Geometry: final body of the model. Coordinates: model frame, mm. Round coordinates to 2 decimals unless told otherwise and drop trailing zeros. Loops run counter-clockwise (first coordinate to the right, second up) from the corner with the lowest first, then second, coordinate; pieces in that order, holes last. Notation, with made-up numbers: M -8.75,-40 L -4.75,-40 A22 cw -4.75,-21 Z; hole C 74.25,28.25 d5. An arc over 180 degrees is marked long. Answer as a JSON object with one key per item and string values.
```python
from build123d import *

# Parameters (mm, degrees)
F0_R     = 4.05
F0_R_2   = 3.200001
F0_R_3   = 3.15
F0_R_4   = 0.75
F0_R_5   = 1
F0_R_6   = 1.1
F1_DEPTH = 2


# Not quite as in the source:
# - ends of sketch curves that miss each other by under 0.0002 mm in the source are joined


with BuildPart() as f1:
    # F0 (on Front) → F1 (new body)
    with BuildSketch(Plane.XZ):
        Polygon((-30.3, -61.250013), (-30.3, -64.250012), (30.300001, -64.250012), (30.300001, 64.250011), (-30.3, 64.250011), align=None)
        with BuildLine():
            ThreePointArc((-23.600001, -59.750013), (-22.7999995588, -59.550011), (-21.9999982215, -59.7500134152))
            Line((-21.9999982215, -59.7500134152), (-21.100001, -59.750013))
            ThreePointArc((-21.100001, -59.750013), (-20.5, -61.2500126379), (-21.1000001998, -62.7500108097))
            Line((-21.1000001998, -62.7500108097), (-21.999999, -62.750012))
            ThreePointArc((-21.999999, -62.750012), (-22.7999995588, -62.950014), (-23.600001, -62.750012))
            Line((-23.600001, -62.750012), (-24.499999, -62.750012))
            ThreePointArc((-24.499999, -62.750012), (-25.1, -61.2500126379), (-24.4999988252, -59.7500141665))
            Line((-24.4999988252, -59.7500141665), (-23.600001, -59.750013))
        make_face(mode=Mode.SUBTRACT)
        with Locations((-19.800001, -47.249931)):
            Circle(F0_R, mode=Mode.SUBTRACT)
        with Locations((-19.800052, -32.249984)):
            Circle(F0_R, mode=Mode.SUBTRACT)
        with Locations((-7.100001, -47.249931)):
            Circle(F0_R, mode=Mode.SUBTRACT)
        with Locations((-7.100052, -32.249984)):
            Circle(F0_R, mode=Mode.SUBTRACT)
        with Locations((-20.549999, -17.249989)):
            Circle(F0_R_2, mode=Mode.SUBTRACT)
        with Locations((-20.549999, -1.999989)):
            Circle(F0_R_3, mode=Mode.SUBTRACT)
        with Locations((-13.8, -22.749991)):
            Circle(F0_R_4, mode=Mode.SUBTRACT)
        with Locations((-7.100052, -17.249986)):
            Circle(F0_R, mode=Mode.SUBTRACT)
        with Locations((-13.200001, -9.499989)):
            Circle(F0_R_5, mode=Mode.SUBTRACT)
        with Locations((-7.100001, -0.749989)):
            Circle(F0_R_2, mode=Mode.SUBTRACT)
        with Locations((7.099976, -47.249957)):
            Circle(F0_R, mode=Mode.SUBTRACT)
        with Locations((7.09995, -32.249928)):
            Circle(F0_R, mode=Mode.SUBTRACT)
        with BuildLine():
            ThreePointArc((22.119986, -59.750023), (22.9199874412, -59.550021), (23.7199887785, -59.7500234152))
            Line((23.7199887785, -59.7500234152), (24.619987, -59.750023))
            ThreePointArc((24.619987, -59.750023), (25.219987, -61.250023), (24.6199863008, -62.7500213341))
            Line((24.6199863008, -62.7500213341), (23.719988, -62.750022))
            ThreePointArc((23.719988, -62.750022), (22.9199874412, -62.950024), (22.119986, -62.750022))
            Line((22.119986, -62.750022), (21.219988, -62.750022))
            ThreePointArc((21.219988, -62.750022), (20.619987, -61.250023), (21.2199901249, -59.7500221189))
            Line((21.2199901249, -59.7500221189), (22.119986, -59.750023))
        make_face(mode=Mode.SUBTRACT)
        with Locations((19.799976, -47.249957)):
            Circle(F0_R, mode=Mode.SUBTRACT)
        with Locations((19.79995, -32.249928)):
            Circle(F0_R, mode=Mode.SUBTRACT)
        with Locations((7.099925, -17.249928)):
            Circle(F0_R, mode=Mode.SUBTRACT)
        with Locations((13.799975, -22.749991)):
            Circle(F0_R_4, mode=Mode.SUBTRACT)
        with Locations((7.100052, -0.749989)):
            Circle(F0_R_2, mode=Mode.SUBTRACT)
        with Locations((13.199999, -9.499989)):
            Circle(F0_R_5, mode=Mode.SUBTRACT)
        with Locations((20.549974, -17.249989)):
            Circle(F0_R_2, mode=Mode.SUBTRACT)
        with Locations((20.549974, -1.999989)):
            Circle(F0_R_3, mode=Mode.SUBTRACT)
        with BuildLine():
            Line((-21.3, 13.150011), (-21.3, 30.750012))
            Line((-21.3, 30.750012), (-21.3, 48.350012))
            ThreePointArc((-21.3, 48.350012), (-21.0363968102, 48.9864088102), (-20.4, 49.250013))
            Line((-20.4, 49.250013), (-19.700001, 49.250013))
            ThreePointArc((-19.700001, 49.250013), (-19.0636041898, 48.9864088102), (-18.8, 48.350012))
            Line((-18.8, 48.350012), (-18.8, 30.750012))
            Line((-18.8, 30.750012), (-18.8, 13.150011))
            ThreePointArc((-18.8, 13.150011), (-19.0636041898, 12.5136141898), (-19.700001, 12.25001))
            Line((-19.700001, 12.25001), (-20.4, 12.250011))
            ThreePointArc((-20.4, 12.250011), (-21.0363968102, 12.5136141898), (-21.3, 13.150011))
        make_face(mode=Mode.SUBTRACT)
        with BuildLine():
            Line((-8.55, 13.150011), (-8.55, 30.750012))
            Line((-8.55, 30.750012), (-8.55, 48.350012))
            ThreePointArc((-8.55, 48.350012), (-8.2863968102, 48.9864088102), (-7.65, 49.250013))
            Line((-7.65, 49.250013), (-6.950001, 49.250013))
            ThreePointArc((-6.950001, 49.250013), (-6.3136041898, 48.9864088102), (-6.05, 48.350012))
            Line((-6.05, 48.350012), (-6.05, 30.750012))
            Line((-6.05, 30.750012), (-6.05, 13.150011))
            ThreePointArc((-6.05, 13.150011), (-6.3136041898, 12.5136141898), (-6.950001, 12.25001))
            Line((-6.950001, 12.25001), (-7.65, 12.250011))
            ThreePointArc((-7.65, 12.250011), (-8.2863968102, 12.5136141898), (-8.55, 13.150011))
        make_face(mode=Mode.SUBTRACT)
        with BuildLine():
            ThreePointArc((-23.600014, 62.750001), (-22.8000125588, 62.950003), (-22.0000112215, 62.7500005848))
            Line((-22.0000112215, 62.7500005848), (-21.100013, 62.750001))
            ThreePointArc((-21.100013, 62.750001), (-20.500013, 61.2500013621), (-21.1000131998, 59.7500031903))
            Line((-21.1000131998, 59.7500031903), (-22.000012, 59.750002))
            ThreePointArc((-22.000012, 59.750002), (-22.8000125588, 59.55), (-23.600014, 59.750002))
            Line((-23.600014, 59.750002), (-24.500012, 59.750002))
            ThreePointArc((-24.500012, 59.750002), (-25.100013, 61.2500013621), (-24.5000093757, 62.7500024055))
            Line((-24.5000093757, 62.7500024055), (-23.600014, 62.750001))
        make_face(mode=Mode.SUBTRACT)
        with Locations((-20.049998, 51.250011)):
            Circle(F0_R_6, mode=Mode.SUBTRACT)
        with BuildLine():
            Line((6.050001, 13.150011), (6.050001, 30.750012))
            Line((6.050001, 30.750012), (6.050001, 48.350012))
            ThreePointArc((6.050001, 48.350012), (6.3136051898, 48.9864088102), (6.950002, 49.250013))
            Line((6.950002, 49.250013), (7.65, 49.250013))
            ThreePointArc((7.65, 49.250013), (8.2863968102, 48.9864088102), (8.550001, 48.350012))
            Line((8.550001, 48.350012), (8.550001, 30.750012))
            Line((8.550001, 30.750012), (8.550001, 13.150011))
            ThreePointArc((8.550001, 13.150011), (8.2863968102, 12.5136141898), (7.65, 12.25001))
            Line((7.65, 12.25001), (6.950002, 12.250011))
            ThreePointArc((6.950002, 12.250011), (6.3136051898, 12.5136141898), (6.050001, 13.150011))
        make_face(mode=Mode.SUBTRACT)
        with BuildLine():
            Line((18.800001, 13.150009), (18.800001, 30.750009))
            Line((18.800001, 30.750009), (18.800001, 48.35001))
            ThreePointArc((18.800001, 48.35001), (19.0636041898, 48.9864068102), (19.700001, 49.250011))
            Line((19.700001, 49.250011), (20.4, 49.25001))
            ThreePointArc((20.4, 49.25001), (21.0363968102, 48.9864068102), (21.300001, 48.35001))
            Line((21.300001, 48.35001), (21.300001, 30.750009))
            Line((21.300001, 30.750009), (21.300001, 13.150009))
            ThreePointArc((21.300001, 13.150009), (21.0363968102, 12.5136121898), (20.4, 12.250008))
            Line((20.4, 12.250008), (19.700001, 12.250008))
            ThreePointArc((19.700001, 12.250008), (19.0636041898, 12.5136121898), (18.800001, 13.150009))
        make_face(mode=Mode.SUBTRACT)
        with Locations((20.050001, 51.250009)):
            Circle(F0_R_6, mode=Mode.SUBTRACT)
        with BuildLine():
            Line((22.119986, 59.750002), (21.219988, 59.750002))
            ThreePointArc((21.219988, 59.750002), (20.619987, 61.2500013621), (21.2199906243, 62.7500024055))
            Line((21.2199906243, 62.7500024055), (22.119986, 62.750001))
            ThreePointArc((22.119986, 62.750001), (22.9199874412, 62.950003), (23.7199887785, 62.7500005848))
            Line((23.7199887785, 62.7500005848), (24.619987, 62.750001))
            ThreePointArc((24.619987, 62.750001), (25.219987, 61.2500013621), (24.6199868002, 59.7500031903))
            Line((24.6199868002, 59.7500031903), (23.719988, 59.750002))
            ThreePointArc((23.719988, 59.750002), (22.9199874412, 59.55), (22.119986, 59.750002))
        make_face(mode=Mode.SUBTRACT)
    extrude(amount=F1_DEPTH)


solid = f1.part
```
1) Cut plane B-B on y = -1. Count the separate pieces of the cut face and the enclosed holes in it, and give its area (3 significant figures).
Geometry results:
{"separate pieces": "1", "enclosed holes": "30", "area": "6,640 mm2"}
2) Cut plane A-A on z = 25. Return the cut outline in (x, y), and give its area (3 significant figures).
Geometry results:
{"outline": "M -30.3,-2 L -21.3,-2 L -21.3,0 L -30.3,0 Z; M -18.8,-2 L -8.55,-2 L -8.55,0 L -18.8,0 Z; M -6.05,-2 L 6.05,-2 L 6.05,0 L -6.05,0 Z; M 8.55,-2 L 18.8,-2 L 18.8,0 L 8.55,0 Z; M 21.3,-2 L 30.3,-2 L 30.3,0 L 21.3,0 Z", "area": "101 mm2"}
3) Line query: probe 1 along Z at (x, y) = (7.5, -1.4); probe 2 along X at (y, z) = (-1.6, 43); probe 3 along Z at (x, y) = (13.2, -0.8). Output: solid intervals per line, ascending.
Geometry results:
{"probe 1": "-64.25 to -51.28, -43.22 to -36.28, -28.22 to -21.28, -13.22 to -3.92, 2.42 to 12.25, 49.25 to 64.25", "probe 2": "-30.3 to -21.3, -18.8 to -8.55, -6.05 to 6.05, 8.55 to 18.8, 21.3 to 30.3", "probe 3": "-64.25 to -23.2, -22.3 to -10.5, -8.5 to 64.25"}
4) Pull-direction query (X, two-part tool) for faces 1 (the face through (0, -2, 1)), 2 (the face through (21.669, -0.986, -35.843)); classes: +X half, -X half, draft (parallel to the pull), parting line (faces both ways), or undercut.
Geometry results:
{"face 1": "draft", "face 2": "undercut"}
